```python
from build123d import *

# Parameters (mm, degrees)
F1_DEPTH  = 1000
F2_W      = 880
F2_H      = 1160
F3_DEPTH  = 795
F5_DEPTH  = 1000
F6_R      = 100
F7_DEPTH  = 60
F8_R      = 35
F9_DEPTH  = 60
F10_R     = 12.5
F11_DEPTH = 590


with BuildPart() as f1:
    # F0 (on Right) → F1 (new body)
    with BuildSketch(Plane.YZ):
        Polygon((710, 1000), (-710, 1000), (-710, -1000), (650, -1000), (650, -520), (710, -520), align=None)
    extrude(amount=-F1_DEPTH)

    # F2 (on face) → F3 (cut)
    with BuildSketch(Plane(origin=(0, 710, 0), x_dir=(-1, 0, 0), z_dir=(0, 1, 0))):
        with Locations((500, 120)):
            Rectangle(F2_W, F2_H)
    extrude(amount=-F3_DEPTH, mode=Mode.SUBTRACT)

    # F4 (on face) → F5 (join, through all)
    with BuildSketch(Plane(origin=(-1000, 0, 0), x_dir=(0, -1, 0), z_dir=(-1, 0, 0))):
        Polygon((-710, 710), (-710, 1000), (-860, 1000), align=None)
    extrude(amount=-F5_DEPTH)

    # F6 (on face) → F7 (join)
    with BuildSketch(Plane(origin=(0, -85, 0), x_dir=(-1, 0, 0), z_dir=(0, 1, 0))):
        with Locations((735.730886, 496.748427)):
            Circle(F6_R)
        with Locations((735.730886, 120)):
            Circle(F6_R)
        with Locations((735.730886, -270.26796)):
            Circle(F6_R)
        with Locations((264.269114, 496.748427)):
            Circle(F6_R)
        with Locations((264.269114, 120)):
            Circle(F6_R)
        with Locations((264.269114, -270.26796)):
            Circle(F6_R)
    extrude(amount=F7_DEPTH)

    # F8 (on face) → F9 (join)
    with BuildSketch(Plane(origin=(0, -25, 0), x_dir=(-1, 0, 0), z_dir=(0, 1, 0))):
        with Locations((735.730886, 496.748427)):
            Circle(F8_R)
        with Locations((735.730886, 120)):
            Circle(F8_R)
        with Locations((735.730886, -270.26796)):
            Circle(F8_R)
        with Locations((264.269114, -270.26796)):
            Circle(F8_R)
        with Locations((264.269114, 120)):
            Circle(F8_R)
        with Locations((264.269114, 496.748427)):
            Circle(F8_R)
    extrude(amount=F9_DEPTH)

    # F10 (on face) → F11 (join)
    with BuildSketch(Plane(origin=(0, 35, 0), x_dir=(-1, 0, 0), z_dir=(0, 1, 0))):
        with Locations((735.730886, 496.748427)):
            Circle(F10_R)
        with Locations((735.730886, 120)):
            Circle(F10_R)
        with Locations((735.730886, -270.26796)):
            Circle(F10_R)
        with Locations((264.269114, -270.26796)):
            Circle(F10_R)
        with Locations((264.269114, 120)):
            Circle(F10_R)
        with Locations((264.269114, 496.748427)):
            Circle(F10_R)
    extrude(amount=F11_DEPTH)


solid = f1.part
```
Design review of the part built by this model. Coordinates are the model's own, in mm. A direction names the side the tool comes from. Give positions to 0.01 mm unless a question says otherwise; leave off trailing zeros. Loops run counter-clockwise (first coordinate to the right, second up) from the corner with the lowest first, then second, coordinate; pieces in that order, holes last. Notation, with made-up numbers: M 28.5,74 L 74.5,74 A36 cw 74.5,108 Z; hole C 27.25,21 d2. An arc over 180 degrees is marked long. Return JSON: item names as keys, results as strings. Group by question number.
Item 1: Tool access review of faces 1 (the flat face through (-494, 318, 700)), 2 (the flat face through (-507, 786.05, 857.03)): name each direction out of +Z, -Z, +X, -X, +Y, -Y from which nothing blocks a thin tool from reaching the whole face with its end or side.
Item 2: We need section B-B (z = -29). Give the boundary of the cut face in (x, y).
Item 3: We need section A-A (x = -400.5). Give the boundary of the cut face in (y, z).
Item 4: For probe 1 along X at (y, z) = (261, -224.5); probe 2 along Z at (x, y) = (-317.5, 84); probe 3 along Z at (x, y) = (-311.5, -34), list the stretches that pass through material, from the lowest coordinate up.
Item 5: We need section C-C (y = 121). Give the boundary of the cut face in (x, z).
Item 6: Mouldability with a two-part tool opening along X and no side actions: class faces 3 (the flat face through (-493, 650, -763)), 4 (the flat face through (-734, -25, 77)) as released by +X, released by -X, zero draft, split by the parting line, or undercut.
Item 7: Insertion check: pin 1 Ø12.5 at (x, z) = (-266, -265) entering from +Y; pin 2 Ø12 at (x, y) = (-798.5, 664.5) entering from -Z. Each pin has a flat end and moves straight along its axis. Give the tip position at first contact, or say it passes through.
Item 8: We need section D-D (z = -626). Give the boundary of the cut face in (x, y), and give its area (3 significant figures).
Output:
{
 "1": {"face 1": "+Y", "face 2": "-Z, +X, -X, +Y"},
 "2": {"outline": "M -1000,-710 L 0,-710 L 0,710 L -60,710 L -60,-85 L -940,-85 L -940,710 L -1000,710 Z"},
 "3": {"outline": "M -710,-1000 L 650,-1000 L 650,-520 L 710,-520 L 710,-460 L -85,-460 L -85,700 L 710,700 L 710,710 L 860,1000 L -710,1000 Z"},
 "4": {"probe 1": "x = -1000 to -940, -60 to 0", "probe 2": "z = -1000 to -460, 700 to 1000", "probe 3": "z = -1000 to -460, -358.41 to -182.12, 31.86 to 208.14, 408.61 to 584.89, 700 to 1000"},
 "5": {"outline": "M -1000,-1000 L 0,-1000 L 0,1000 L -1000,1000 Z; C -735.73,-270.27 d25; C -735.73,120 d25; C -735.73,496.75 d25; C -264.27,-270.27 d25; C -264.27,120 d25; C -264.27,496.75 d25; hole M -940,-460 L -60,-460 L -60,700 L -940,700 Z"},
 "6": {"face 3": "zero draft", "face 4": "undercut"},
 "7": {"pin 1": "stops at y = 625", "pin 2": "stops at z = -520"},
 "8": {"outline": "M -1000,-710 L 0,-710 L 0,650 L -1000,650 Z", "area": "1,360,000 mm^2"}
}
